CAD build for the part. Positions are in the model's coordinates, mm. A direction names the side the tool comes from. Coordinates: 2 decimals unless noted, no trailing zeros. Write each loop counter-clockwise with the first axis right and the second up, starting at its lowest first coordinate (ties: lowest second). Pieces come first, ordered by that corner, then holes. Notation, with made-up numbers: (25.5, 23) - (29.5, 23) arc R33 ccw to (29.5, 60) - close; hole circle Ø2 at (40, 17.5). An arc over 180 degrees is marked (long way). Answer in a Markdown table with one row per item. Add a question column.
Q1. Two-plate mould, pull along Y, no slides. Class faces 1 (the cylindrical face through (-0.37, -1.65, 2.01)), 2 (the flat face through (0, 0, 3)), 3 (the cylindrical face through (-7.493, 0.33, 1.479)): +Y half, -Y half, draft (parallel to the pull), parting line (faces both ways), or undercut.
Q2. Drill centre lines: line 1 along Y through (x, z) = (0, 1.75); line 2 along X through (y, z) = (0.5, 2.65); line 3 along Y through (x, z) = (1.5, 2.3). Where is each one in solid material? Low to high. Write a range as from..to.
Q3. 3-axis set-ups, long thin cutter, end or side, ignore diameter. For faces 4 (the cylindrical face through (-0.439, -1.978, 2.007)), 5 (the flat face through (0, 0, 0)): which of +Z, -Z, +X, -X, +Y, -Y reach the whole face in a straight line?
Q4. Band-saw the part on A-A (x = 0). List the corners of the cut face in (y, z), and give its area (3 significant figures).
Q5. Pin check, flat tip, straight feed: pin 1 (1.5 mm diameter, centred on y = -2.5, z = 2, fed in from -X). Stop position of the tip, or through.
Q6. Band-saw the part on D-D (x = -6). List the corners of the cut face in (y, z), and give its area (3 significant figures).
Q7. Band-saw the part on C-C (z = 1.2). List the corners of the cut face in (x, y).
```python
from build123d import *

# Parameters (mm, degrees)
F0_R     = 7.5
F0_R_2   = 2.0257797654
F0_R_3   = 1.6893187084
F1_DEPTH = 3
F2_R     = 2.0257797654
F2_R_2   = 1.6893187084
F3_DEPTH = 1.5
F4_R     = 0.5


with BuildPart() as f1:
    # F0 (on Top) → F1 (new body)
    with BuildSketch(Plane.XY):
        Circle(F0_R)
        Circle(F0_R_2, mode=Mode.SUBTRACT)
        Circle(F0_R_2)
        Circle(F0_R_3, mode=Mode.SUBTRACT)
        Circle(F0_R_3)
    extrude(amount=F1_DEPTH)

    # F2 (on face) → F3 (cut)
    with BuildSketch(Plane.XY.offset(3)):
        Circle(F2_R)
        Circle(F2_R_2, mode=Mode.SUBTRACT)
    extrude(amount=-F3_DEPTH, mode=Mode.SUBTRACT)

    # F4
    f4_edges = [f1.edges().sort_by_distance(p)[0] for p in [
        (-1.689319, 0, 3),
        (-2.02578, 0, 3),
    ]]
    fillet(f4_edges, radius=F4_R)


solid = f1.part
```
Checked values:
| question | item | result |
|---|---|---|
| 1 | face 1 | undercut |
| 1 | face 2 | draft |
| 1 | face 3 | parting line |
| 2 | line 1 | y = -7.5..-2.03, -1.69..1.69, 2.03..7.5 |
| 2 | line 2 | x = -7.48..-1.99, -1.59..1.59, 1.99..7.48 |
| 2 | line 3 | y = -7.35..-1.36, -0.78..0.78, 1.36..7.35 |
| 3 | face 4 | +Z |
| 3 | face 5 | -Z, +X, -X, +Y, -Y |
| 4 | outline | (-7.5, 0) - (7.5, 0) - (7.5, 3) - (2.53, 3) arc R0.5 ccw to (2.03, 2.5) - (2.03, 1.5) - (1.69, 1.5) - (1.69, 2.5) arc R0.5 ccw to (1.19, 3) - (-1.19, 3) arc R0.5 ccw to (-1.69, 2.5) - (-1.69, 1.5) - (-2.03, 1.5) - (-2.03, 2.5) arc R0.5 ccw to (-2.53, 3) - (-7.5, 3) - close |
| 4 | area | 43.8 mm² |
| 5 | pin 1 | stops at x = -7.29 |
| 6 | outline | (-4.5, 0) - (4.5, 0) - (4.5, 3) - (-4.5, 3) - close |
| 6 | area | 27.0 mm² |
| 7 | outline | circle Ø15 at (0, 0) |
